Read the model definition and answer for the solid it produces. Units are mm, in the model's axes. A direction names the side the tool comes from. Round coordinates to 2 decimals unless told otherwise and drop trailing zeros. Write each loop counter-clockwise with the first axis right and the second up, starting at its lowest first coordinate (ties: lowest second). Pieces come first, ordered by that corner, then holes. Notation, with made-up numbers: (49, -22) - (105, -22) arc R17 cw to (105, -4) - close; hole circle Ø10 at (27.5, 35.25). An arc over 180 degrees is marked (long way). Use one line per item in the form item = value. Start each with the question number.
1) For a pull along X with two mould halves and no side action, classify faces 3 (the face through (6, 0, 2)), 4 (the face through (-0.04, -17.22, -9.82)), 5 (the face through (-10.316, -7.91, 0.986)) as released by +X, released by -X, zero draft, split by the parting line, or undercut.
2) Consider line 1 along Y through (x, z) = (0, -3.25); line 2 along X through (y, z) = (-1.5, -8); line 3 along Z through (x, y) = (-17.5, -13). Determine where each line is inside the solid, lowest interval first. Write a range as from..to.
3) The part is cut by section C-C, the plane z = -58. Give the vertices of the cut face in (x, y).
4) Each of these flat-tipped pins is pushed along its axis until it touches: pin 1 (12 mm diameter, centred on x = -17, z = -69.5, fed in from -Y); pin 2 (3 mm diameter, centred on x = 0, y = -17.5, fed in from +Z); pin 3 (3 mm diameter, centred on x = 12.5, y = 13, fed in from +Z). Where does it stop, or does it pass through?
5) The part is cut by section B-B, the plane x = -6.5. Give the vertices of the cut face in (y, z), plus the area to 3 significant figures.
6) The part is cut by section A-A, the plane z = -3. Give the vertices of the cut face in (x, y).
7) The part is cut by section D-D, the plane y = -9. Give the vertices of the cut face in (x, z), plus the area to 3 significant figures.
8) For faces 1 (the face through (10.413, 11.521, -12.325)), 2 (the face through (0, 0, 29)), determine the directions among +Z, -Z, +X, -X, +Y, -Y from which every point of the face is accessible in a straight line to the end or side of a thin tool.
from build123d import *

# Parameters (mm, degrees)
SKETCH1_R                   = 22.5
BOSS_EXTRUDE1_DEPTH         = 131.9
SKETCH2_R                   = 13
BOSS_EXTRUDE2_DEPTH         = 2
SKETCH3_R                   = 5
BOSS_EXTRUDE3_DEPTH         = 27
M4_TAPPED_HOLE1_D           = 3.3
M4_TAPPED_HOLE1_DEPTH       = 9
M4_TAPPED_HOLE1_CSINK_D     = 4.05
M4_TAPPED_HOLE1_CSINK_ANGLE = 90
M4_TAPPED_HOLE1_TIP         = 0.991420021
SKETCH7_R                   = 2
CUT_EXTRUDE1_DEPTH          = 25


with BuildPart() as part:
    # Sketch1 → Boss-Extrude1 (new body)
    with BuildSketch(Plane.XY):
        Circle(SKETCH1_R)
    extrude(amount=-BOSS_EXTRUDE1_DEPTH)

    # Sketch2 → Boss-Extrude2 (add)
    with BuildSketch(Plane.XY):
        Circle(SKETCH2_R)
    extrude(amount=BOSS_EXTRUDE2_DEPTH)

    # Sketch3 → Boss-Extrude3 (add)
    with BuildSketch(Plane.XY.offset(2)):
        Circle(SKETCH3_R)
    extrude(amount=BOSS_EXTRUDE3_DEPTH)

    # M4 Tapped Hole1
    with Locations(Plane.XY):
        with Locations((0, 17.5), (-17.5, 0), (0, -17.5), (17.5, 0)):
            CounterSinkHole(M4_TAPPED_HOLE1_D / 2, M4_TAPPED_HOLE1_CSINK_D / 2, depth=M4_TAPPED_HOLE1_DEPTH, counter_sink_angle=M4_TAPPED_HOLE1_CSINK_ANGLE)
            with Locations((0, 0, -(M4_TAPPED_HOLE1_DEPTH + M4_TAPPED_HOLE1_TIP / 2))):  # 118° drill point
                Cone(0, M4_TAPPED_HOLE1_D / 2, M4_TAPPED_HOLE1_TIP, mode=Mode.SUBTRACT)

    # Sketch7 → Cut-Extrude1 (cut)
    with BuildSketch(Plane.XY):
        with Locations((-12, 12.737739203)):
            Circle(SKETCH7_R)
        with Locations((12, 12.737739203)):
            Circle(SKETCH7_R)
    extrude(amount=-CUT_EXTRUDE1_DEPTH, mode=Mode.SUBTRACT)


solid = part.part
Geometry results:
q1.face_3 = zero draft
q1.face_4 = undercut
q1.face_5 = split by the parting line
q2.line_1 = -22.5..-19.15, -15.85..15.85, 19.15..22.5
q2.line_2 = -22.45..-18.19, -16.81..16.81, 18.19..22.45
q2.line_3 = -131.9..0
q3.outline = circle Ø45 at (0, 0)
q4.pin_1 = -19.63
q4.pin_2 = -9.09
q4.pin_3 = 0
q5.outline = (-21.54, -131.9) - (21.54, -131.9) - (21.54, 0) - (11.26, 0) - (11.26, 2) - (-11.26, 2) - (-11.26, 0) - (-21.54, 0) - close
q5.area = 5,730 mm2
q6.outline = circle Ø45 at (0, 0); hole circle Ø3.3 at (-17.5, 0); hole circle Ø4 at (-12, 12.74); hole circle Ø3.3 at (0, -17.5); hole circle Ø3.3 at (0, 17.5); hole circle Ø4 at (12, 12.74); hole circle Ø3.3 at (17.5, 0)
q7.outline = (-20.62, -131.9) - (20.62, -131.9) - (20.62, 0) - (9.38, 0) - (9.38, 2) - (-9.38, 2) - (-9.38, 0) - (-20.62, 0) - close
q7.area = 5,480 mm2
q8.face_1 = +Z
q8.face_2 = +Z, +X, -X, +Y, -Y
